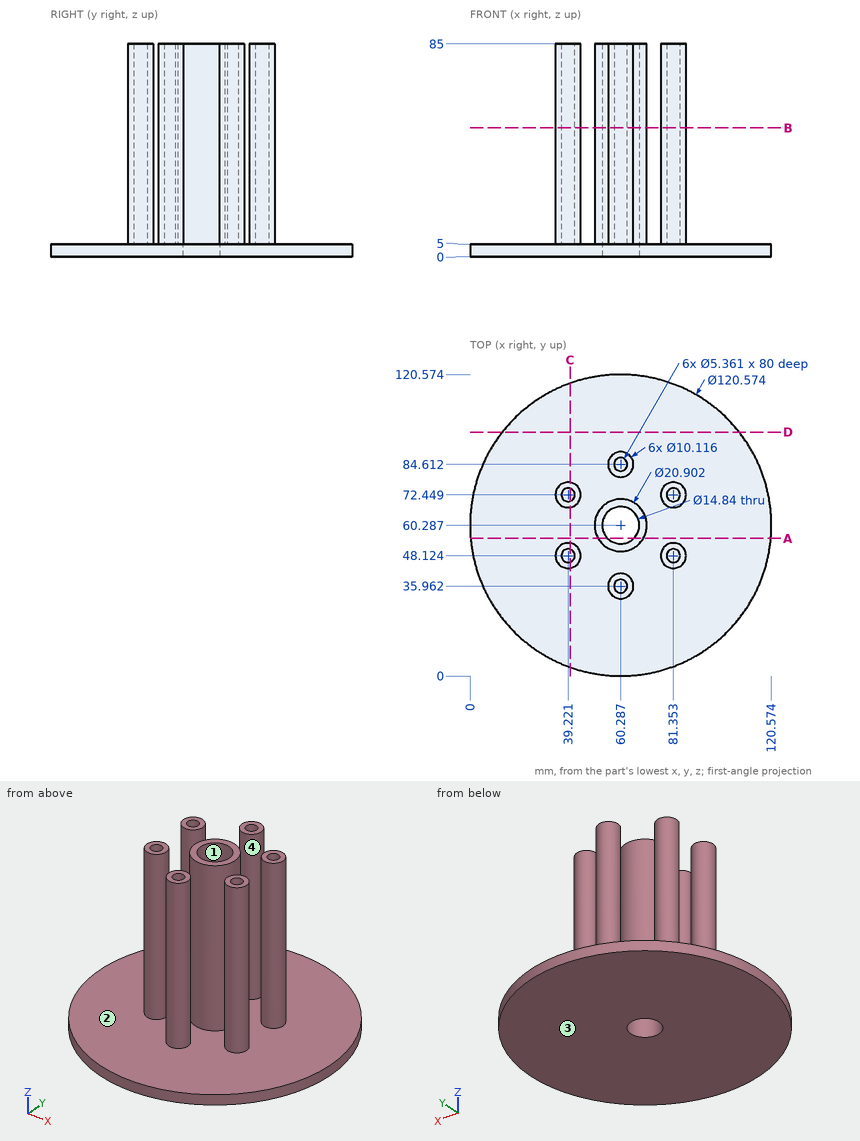
Design review of the part shown in the three views and the two pictorial views. Dimensions are in mm from the part's minimum x, y and z. A direction names the side the tool comes from. Round coordinates to 2 decimals unless told otherwise and drop trailing zeros. Loops run counter-clockwise (first coordinate to the right, second up) from the corner with the lowest first, then second, coordinate; pieces in that order, holes last.
1) Consider section A-A on y = 55. State the section outline as (x, z) points, then the cut area to 3 significant figures.
Values follow:
outline: (0.23, 0) - (55.08, 0) - (55.08, 85) - (51.27, 85) - (51.27, 5) - (0.23, 5) - close; (65.49, 0) - (120.34, 0) - (120.34, 5) - (69.3, 5) - (69.3, 85) - (65.49, 85) - close
area: 1,160 mm2
2) Consider section D-D on y = 97.5. State the section outline as (x, z) points (1 decimal).
Values follow:
outline: (12.9, 0) - (107.7, 0) - (107.7, 5) - (12.9, 5) - close
3) The part is to be moulded in two halves that separate along Y. For the marked faces 3 and 4, say which applies: pulls with the +Y half, pulls with the -Y half, needs draft (parallel to the pull), parting line crosses it, or undercut.
Values follow:
face 3: needs draft
face 4: undercut
4) Wall thickness on line 1 along X through (y, z) = (46, 69.5) (1 decimal); line 2 along Z through (x, y) = (83, 110); line 3 along Y through (x, z) = (66.5, 28.5) (1 decimal): over which ranges is each line inside the solid? List them lowest first.
Values follow:
line 1: x = 34.6 to 37.6, 40.9 to 43.8, 76.8 to 79.7, 83 to 85.9
line 2: z = 0 to 5
line 3: y = 51.9 to 56.2, 64.3 to 68.7
5) Consider section B-B on z = 51.5. Give the number of separate pieces and of enclosed holes in the cut face, then the cut area to 3 significant figures.
Values follow:
separate pieces: 7
enclosed holes: 7
area: 517 mm2
6) Tool access review of the marked faces 1 and 2: name each direction out of +Z, -Z, +X, -X, +Y, -Y from which nothing blocks a thin tool from reaching the whole face with its end or side.
Values follow:
face 1: +Z, -Z
face 2: +Z
7) Consider section C-C on x = 40. State the section outline as (y, z) points (1 decimal).
Values follow:
outline: (3.5, 0) - (117.1, 0) - (117.1, 5) - (77.4, 5) - (77.4, 85) - (75, 85) - (75, 5) - (69.9, 5) - (69.9, 85) - (67.5, 85) - (67.5, 5) - (53.1, 5) - (53.1, 85) - (50.7, 85) - (50.7, 5) - (45.6, 5) - (45.6, 85) - (43.1, 85) - (43.1, 5) - (3.5, 5) - close
8) Clearance check with flat-ended pins moving along their axes: P1, Ø3, axis at x = 39.22, y = 72.45, coming from the +Z side; P2, Ø2, axis at x = 46, z = 28.5, coming from the +Y side; P3, Ø6, axis at x = 59, y = 85, coming from the +Z side; P4, Ø10, axis at x = 37.5, z = 61.5, coming from the -Y side. State where each tip first meets the part, or that it passes through.
Values follow:
P1: stops at z = 5
P2: passes through
P3: stops at z = 85
P4: stops at y = 43.07
